Autodesk Inventor part; units mm, degrees
ref_plane "YZ Plane" through (0, 0, 0) normal (1, 0, 0) x (0, 1, 0)
ref_plane "XZ Plane" through (0, 0, 0) normal (0, 1, 0) x (-1, 0, 0)
ref_plane "XY Plane" through (0, 0, 0) normal (0, 0, 1) x (1, 0, 0)
ref_plane "Arbeitsebene1" through (21.5439, 0, 2.0695) normal (0, 0, -1) x (-1, 0, 0)
sketch "Skizze1" plane through (21.5439, 0, 2.0695) normal (0, 0, -1) x (-1, 0, 0)
  line L0 (-25, -25) -> (25, -25)
  line L1 (25, -25) -> (25, 25)
  line L2 (25, 25) -> (-25, 25)
  line L3 (-25, 25) -> (-25, -25)
  line L4 (-25, -25) -> (25, 25) construction
  line L5 (25, -25) -> (-25, 25) construction
  line L6 (-17, -17) -> (17, -17)
  line L7 (17, -17) -> (17, 17)
  line L8 (17, 17) -> (-17, 17)
  line L9 (-17, 17) -> (-17, -17)
  line L10 (-17, -17) -> (17, 17) construction
  line L11 (17, -17) -> (-17, 17) construction
  point P0 (21.5439, 0)
  point P1 (0, 0)
  point P2 (0, 0)
  dimension "d0" = 50
  dimension "d1" = 50
  dimension "d2" = 34
  dimension "d3" = 34
extrude "Extrusion1" add sketch "Skizze1" along normal blind 5
sketch "Skizze2" plane through (21.5439, 0, -2.9305) normal (0, 0, -1) x (-1, 0, 0)
  line L0 (21, 17) -> (21, -17)
  line L1 (25, -25) -> (25, 25)
  line L2 (25, 25) -> (-25, 25)
  line L3 (-25, 25) -> (-25, -25)
  line L4 (-25, -25) -> (25, -25)
  line L5 (-17, -17) -> (-17, 17)
  line L6 (-17, 17) -> (17, 17)
  line L7 (17, 17) -> (17, -17)
  line L8 (17, -17) -> (-17, -17)
  line L9 (20.5, -20.5) -> (-20.5, -20.5)
  line L10 (-20.5, -20.5) -> (-20.5, 20.5)
  line L11 (-20.5, 20.5) -> (20.5, 20.5)
  line L12 (20.5, 20.5) -> (20.5, -20.5)
  line L13 (20.5, -20.5) -> (-20.5, 20.5) construction
  line L14 (-20.5, -20.5) -> (20.5, 20.5) construction
  point P0 (21.5439, 0)
  point P1 (0, 0)
  point P2 (-14.5, 20.5)
  point P3 (-20.5, 14.5)
  dimension "d6" = 41
  dimension "d7" = 41
  dimension "d_pin" = 14.5
  dimension "d10" = 14.5
hole "Bohrung1" at (36.0439, 20.5, -2.9305) at (42.0439, 14.5, -2.9305) at (42.0439, 20.5, -2.9305) direction (0, 0, 1) diameter 4.8 end through all
ref_plane "Arbeitsebene2" through (21.5439, -25, 2.0695) normal (1, 0, 0) x (0, 0, -1)
ref_plane "Arbeitsebene3" through (-3.4561, 0, 2.0695) normal (0, -1, 0) x (1, 0, 0)
pattern_circular "Runde Anordnung1" count 4 over 360 about axis through (21.5439, 0, 2.0695) along (0, 0, 1) of "Bohrung1"
fillet "Rundung1" radius 2 8 edges at (38.5439, 17, -0.4305) (38.5439, -17, -0.4305) (4.5439, -17, -0.4305) (4.5439, 17, -0.4305) (-3.4561, 25, -0.4305) (-3.4561, -25, -0.4305) (46.5439, -25, -0.4305) (46.5439, 25, -0.4305)
properties part number "10_Base_v4"
Work out the finished part from the listing and answer in its coordinate system (mm). A direction names the side the tool comes from. Round coordinates to 2 decimals unless told otherwise and drop trailing zeros. Write each loop counter-clockwise with the first axis right and the second up, starting at its lowest first coordinate (ties: lowest second). Pieces come first, ordered by that corner, then holes. Notation, with made-up numbers: (38.5, -15) - (49.5, -15) arc R14 cw to (49.5, -3) - close; hole circle Ø11 at (3.25, 38.5). An arc over 180 degrees is marked (long way). Return JSON: item names as keys, results as strings. Group by question number.
Q1. The part is cut by section A-A on x = 22. Write down the section's boundary in (y, z), then the cut area to 3 significant figures.
Q2. For faces 1 (the flat face through (21, 17, 0)), 2 (the flat face through (-3.456, 0, 0)), determine the directions among +Z, -Z, +X, -X, +Y, -Y from which every point of the face is accessible in a straight line to the end or side of a thin tool.
Q3. Find the intervals of material crossed by L1, parallel to X at y = 20.5, z = 0.35; L2, parallel to X at y = 14.5, z = -1.55; L3, parallel to Y at x = -1, z = -0.2, in increasing order.
Q4. The part is cut by section D-D on z = 1.5. Count the separate pieces of the cut face and the enclosed holes in it, then the cut area to 3 significant figures.
Q5. The part is cut by section C-C on y = 20.5. Write down the section's boundary in (x, z), then the cut area to 3 significant figures.
Q6. The part is cut by section B-B on y = 9.5. Write down the section's boundary in (x, z).
Q7. This flat-tipped pin is pushed along its axis until it touches: pin 1 Ø7.5 at (x, y) = (1.04, 14.5) entering from +Z. Where does it stop, or does it pass through?
Q8. The mould has two halves that part along X. Classify faces 3 (the cylindrical face through (-2.886, 24.399, -0.466)), 4 (the cylindrical face through (37.97, -16.4, -0.47)), 5 (the flat face through (39, 6, -2.93)): released by +X, released by -X, zero draft, split by the parting line, or undercut.
Solved:
{
 "1": {"outline": "(-25, -2.93) - (-17, -2.93) - (-17, 2.07) - (-25, 2.07) - close; (17, -2.93) - (25, -2.93) - (25, 2.07) - (17, 2.07) - close", "area": "80.0 mm²"},
 "2": {"face 1": "+Z, -Z", "face 2": "+Z, -Z, -X, +Y, -Y"},
 "3": {"L1": "-3.46 to -1.36, 3.44 to 4.64, 9.44 to 33.64, 38.44 to 39.64, 44.44 to 46.54", "L2": "-3.46 to -1.36, 3.44 to 4.54, 38.54 to 39.64, 44.44 to 46.54", "L3": "-25 to -21.76, -19.24 to -15.76, -13.24 to 13.24, 15.76 to 19.24, 21.76 to 25"},
 "4": {"separate pieces": "1", "enclosed holes": "13", "area": "1,130 mm²"},
 "5": {"outline": "(-3.46, -2.93) - (-1.36, -2.93) - (-1.36, 2.07) - (-3.46, 2.07) - close; (3.44, -2.93) - (4.64, -2.93) - (4.64, 2.07) - (3.44, 2.07) - close; (9.44, -2.93) - (33.64, -2.93) - (33.64, 2.07) - (9.44, 2.07) - close; (38.44, -2.93) - (39.64, -2.93) - (39.64, 2.07) - (38.44, 2.07) - close; (44.44, -2.93) - (46.54, -2.93) - (46.54, 2.07) - (44.44, 2.07) - close", "area": "154 mm²"},
 "6": {"outline": "(-3.46, -2.93) - (4.54, -2.93) - (4.54, 2.07) - (-3.46, 2.07) - close; (38.54, -2.93) - (46.54, -2.93) - (46.54, 2.07) - (38.54, 2.07) - close"},
 "7": {"pin 1": "z = 2.07"},
 "8": {"face 3": "released by -X", "face 4": "undercut", "face 5": "zero draft"}
}
